The listing builds one solid part. Answer for the finished solid, in the listing's coordinates (mm). A direction names the side the tool comes from. Round coordinates to 2 decimals unless told otherwise and drop trailing zeros. Order: outer loops, then holes, each group sorted by start corner. A loop starts at its lowest first (then second) coordinate and runs counter-clockwise, first axis right, second up. Notation, with made-up numbers: M 75.5,0.25 L 122.5,0.25 A31 ccw 122.5,35.25 Z; hole C 11,-3 d5. An arc over 180 degrees is marked long. Write item = value, one per line. Start each with the question number.
(1) For a pull along X with two mould halves and no side action, classify faces 4 (the face through (0, 4, 1)), 5 (the face through (-5.43, 6.25, 1.63)), 6 (the face through (-9, 4, 2)), 7 (the face through (-18, 4, 1)) as released by +X, released by -X, zero draft, split by the parting line, or undercut.
(2) A cutting plane is placed at D-D, the plane x = -2.5. Determine the outline of the cut face in (y, z), and give its area (3 significant figures).
(3) Which of the six approach directions +Z, -Z, +X, -X, +Y, -Y give full straight-line access (tool end or side, diameter ignored) to faces 1 (the face through (-13, 0, 1)), 2 (the face through (-6, 5, 1.25)), 3 (the face through (-7, 2, 1))?
(4) A cutting plane is placed at A-A, the plane z = 0.2. Determine the outline of the cut face in (x, y), and give its area (3 significant figures).
(5) Straight lines are drawn through the part: probe 1 along Y at (x, z) = (-14, 1.95); probe 2 along X at (y, z) = (4, 1.95); probe 3 along X at (y, z) = (1.25, 1.9). For each, find the intervals that lie inside material, in ascending order. Write a range as from..to.
(6) A cutting plane is placed at C-C, the plane y = 4. Determine the outline of the cut face in (x, z), and give its area (3 significant figures).
(7) Each of these flat-tipped pins is pushed along its axis until it touches: pin 1 (4 mm diameter, centred on x = -14, y = 4, fed in from -Z); pin 2 (1.9 mm diameter, centred on x = -5.5, y = 3, fed in from +Z). Where does it stop, or does it pass through?
(8) A cutting plane is placed at B-B, the plane x = -14. Determine the outline of the cut face in (y, z).
Autodesk Inventor part; units mm, degrees
ref_plane "YZ Plane" through (0, 0, 0) normal (1, 0, 0) x (0, 1, 0)
ref_plane "XZ Plane" through (0, 0, 0) normal (0, 1, 0) x (-1, 0, 0)
ref_plane "XY Plane" through (0, 0, 0) normal (0, 0, 1) x (1, 0, 0)
sketch "Skizze1" plane through (0, 0, 0) normal (0, 0, 1) x (1, 0, 0)
  line L0 (-21.6, 0) -> (3.6, 0)
  line L1 (0, -1.6) -> (0, 9.6)
  line L2 (0, 0) -> (-18, 0)
  line L3 (-18, 0) -> (-18, 8)
  line L4 (-18, 8) -> (0, 8)
  line L5 (0, 8) -> (0, 0)
  dimension "d0" = 8
  dimension "d1" = 18
extrude "Extrusion1" add sketch "Skizze1" along normal blind 2
sketch "Skizze2" plane through (0, 0, 2) normal (0, 0, 1) x (1, 0, 0)
  line L0 (-18, 0) -> (0, 0)
  line L1 (0, 0) -> (0, 8)
  point P0 (-5.5, 3)
  dimension "d4" = 5.5
  dimension "d5" = 3
hole "Bohrung1" at (-5.5, 3, 2) direction (0, 0, -1) diameter 3 depth 8 tip angle 118
sketch "Skizze3" plane through (0, 0, 2) normal (0, 0, 1) x (1, 0, 0)
  circle A0 centre (-5.5, 3) radius 1.5
  line L0 (-18, 0) -> (0, 0)
  arc A1 (-2.25, 3) -> (-8.75, 3) centre (-5.5, 3) ccw
  line L1 (-8.75, 3) -> (-8.75, 0)
  line L2 (-2.25, 3) -> (-2.25, 0)
  dimension "d13" = 6.5
extrude "Extrusion2" cut sketch "Skizze3" against normal blind 0.75
sketch "Skizze4" plane through (0, 0, 1.25) normal (0, 0, 1) x (1, 0, 0)
  circle A0 centre (-5.5, 3) radius 1.5
  line L0 (-2.25, 0) -> (-8.75, 0)
  line L1 (-7, 3) -> (-7, 0)
  line L2 (-4, 3) -> (-4, 0)
  point P0 (0, 0)
extrude "Extrusion3" cut sketch "Skizze4" against normal through all contours L2 L0 L1 A0
sketch "Skizze5" plane through (0, 0, 0) normal (0, 0, -1) x (-1, 0, 0)
  line L0 (7, 0) -> (18, 0)
  line L1 (18, 0) -> (18, 8)
  arc A0 (8.75, 3) -> (2.25, 3) centre (5.5, 3) ccw
  point P0 (14, 4)
  dimension "d18" = 4
  dimension "d19" = 4
hole "Bohrung2" at (-14, 4, 0) direction (0, 0, 1) diameter 3.4 end through all countersink diameter 6.9 countersink angle 90
properties part number "13_1087_036"
Reported:
q1.face_4 = released by +X
q1.face_5 = undercut
q1.face_6 = zero draft
q1.face_7 = released by -X
q2.outline = M 0,0 L 8,0 L 8,2 L 4.25,2 L 4.25,1.25 L 0,1.25 Z
q2.area = 12.8 mm²
q3.face_1 = +Z, -Z, +X, -X, -Y
q3.face_2 = +Z, -Y
q3.face_3 = +Z, -Z, -Y
q4.outline = M -18,0 L -7,0 L -7,3 A1.5 cw -4,3 L -4,0 L 0,0 L 0,8 L -18,8 Z; hole C -14,4 d6.5
q4.area = 98.3 mm²
q5.probe_1 = 0..2.3, 5.7..8
q5.probe_2 = -18..-15.7, -12.3..-8.59, -2.41..0
q5.probe_3 = -18..-8.75, -2.25..0
q6.outline = M -18,0 L -17.45,0 L -15.7,1.75 L -15.7,2 L -18,2 Z; M -12.3,1.75 L -10.55,0 L -6.62,0 L -6.62,1.25 L -8.59,1.25 L -8.59,2 L -12.3,2 Z; M -4.38,0 L 0,0 L 0,2 L -2.41,2 L -2.41,1.25 L -4.38,1.25 Z
q6.area = 18.7 mm²
q7.pin_1 = 1.45
q7.pin_2 = through
q8.outline = M 0,0 L 0.55,0 L 2.3,1.75 L 2.3,2 L 0,2 Z; M 5.7,1.75 L 7.45,0 L 8,0 L 8,2 L 5.7,2 Z
